Read the model definition and answer for the solid it produces. Units are mm, in the model's axes. Coordinates: 2 decimals unless noted, no trailing zeros. Write each loop counter-clockwise with the first axis right and the second up, starting at its lowest first coordinate (ties: lowest second). Pieces come first, ordered by that corner, then holes. Notation, with made-up numbers: (8.25, 60) - (16.25, 60) arc R30 ccw to (16.25, 89) - close; hole circle Ø6 at (19, -12.75). An arc over 180 degrees is marked (long way). Use a Markdown table: item, result.
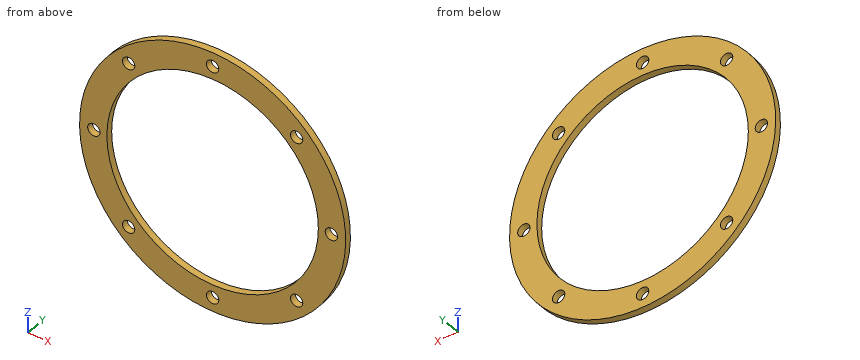
from build123d import *

# Parameters (mm, degrees)
SKETCH1_R           = 28
SKETCH1_R_2         = 22.25
BOSS_EXTRUDE1_DEPTH = 1.4
CIRPATTERN1_COUNT   = 8


with BuildPart() as part:
    # Sketch1 → Boss-Extrude1 (new body)
    with BuildSketch(Plane(origin=(0, 0, 0), x_dir=(1, 0, 0), z_dir=(0, 1, 0))):
        with Locations(Location((0, 0, 0), (0, 0, 270))):
            Circle(SKETCH1_R)
        with Locations(Location((0, 0, 0), (0, 0, 270))):
            Circle(SKETCH1_R_2, mode=Mode.SUBTRACT)
    extrude(amount=BOSS_EXTRUDE1_DEPTH)

    # Sketch4 → M2 Clearance Hole1 (revolve, cut)
    with BuildSketch(Plane(origin=(0, 1.4, -25), x_dir=(0, 0, 1), z_dir=(1, 0, 0))):
        Polygon((0, 0), (0, 17.799118805), (1.3, 17.018), (1.3, 0), align=None)
    m2_clearance_hole1 = revolve(axis=Axis((0, 7.75, -25), (0, -1, 0)), mode=Mode.SUBTRACT)

    # CirPattern1: M2 Clearance Hole1 ×8 about axis
    cirpattern1_axis = Axis((0, 0, 0), (0, 1, 0))
    for i in range(1, CIRPATTERN1_COUNT):
        add(m2_clearance_hole1.rotate(cirpattern1_axis, i * 360 / CIRPATTERN1_COUNT), mode=Mode.SUBTRACT)


solid = part.part
(1) A cutting plane is placed at B-B, the plane x = 0. Write down the section's boundary in (y, z).
Report:
| item | result |
|---|---|
| outline | (0, -28) - (1.4, -28) - (1.4, -26.3) - (0, -26.3) - close; (0, -23.7) - (1.4, -23.7) - (1.4, -22.25) - (0, -22.25) - close; (0, 22.25) - (1.4, 22.25) - (1.4, 23.7) - (0, 23.7) - close; (0, 26.3) - (1.4, 26.3) - (1.4, 28) - (0, 28) - close |
(2) A cutting plane is placed at A-A, the plane z = 0. Write down the section's boundary in (x, y).
Report:
| item | result |
|---|---|
| outline | (-28, 0) - (-26.3, 0) - (-26.3, 1.4) - (-28, 1.4) - close; (-23.7, 0) - (-22.25, 0) - (-22.25, 1.4) - (-23.7, 1.4) - close; (22.25, 0) - (23.7, 0) - (23.7, 1.4) - (22.25, 1.4) - close; (26.3, 0) - (28, 0) - (28, 1.4) - (26.3, 1.4) - close |
(3) A cutting plane is placed at C-C, the plane x = 25. Write down the section's boundary in (y, z).
Report:
| item | result |
|---|---|
| outline | (0, -12.61) - (1.4, -12.61) - (1.4, -1.3) - (0, -1.3) - close; (0, 1.3) - (1.4, 1.3) - (1.4, 12.61) - (0, 12.61) - close |
(4) Straight lines are drawn through the part: L1, parallel to Z at x = 16.5, y = 1.2; L2, parallel to X at y = 0.65, z = -18; L3, parallel to X at y = 0.25, z = 1. For each, find the intervals that lie inside material, in ascending order.
Report:
| item | result |
|---|---|
| L1 | z = -22.62 to -18.23, -17.13 to -14.93, 14.93 to 17.13, 18.23 to 22.62 |
| L2 | x = -21.45 to -18.94, -16.42 to -13.08, 13.08 to 16.42, 18.94 to 21.45 |
| L3 | x = -27.98 to -25.83, -24.17 to -22.23, 22.23 to 24.17, 25.83 to 27.98 |
(5) A cutting plane is placed at D-D, the plane y = 0.8. Count the separate pieces of the cut face and the enclosed holes in it, and give its area (3 significant figures).
Report:
| item | result |
|---|---|
| separate pieces | 1 |
| enclosed holes | 9 |
| area | 865 mm² |
